from build123d import *

# Parameters (mm, degrees)
BOSS_EXTRUDE1_DEPTH = 70
SKETCH2_R           = 10
CUT_EXTRUDE1_DEPTH  = 20
SKETCH3_R           = 20
CUT_EXTRUDE2_DEPTH  = 71


with BuildPart() as part:
    # Sketch1 → Boss-Extrude1 (new body)
    with BuildSketch(Plane(origin=(0, 0, 0), x_dir=(1, 0, 0), z_dir=(0, 1, 0))):
        with BuildLine():
            Line((0, 100), (600, 100))
            ThreePointArc((600, 100), (700, 0), (600, -100))
            Line((600, -100), (0, -100))
            ThreePointArc((0, -100), (-100, 0), (0, 100))
        make_face()
    extrude(amount=BOSS_EXTRUDE1_DEPTH)

    # Sketch2 → Cut-Extrude1 (cut)
    with BuildSketch(Plane(origin=(0, 70, 0), x_dir=(1, 0, 0), z_dir=(0, 1, 0))):
        Circle(SKETCH2_R)
    extrude(amount=-CUT_EXTRUDE1_DEPTH, mode=Mode.SUBTRACT)

    # Sketch3 → Cut-Extrude2 (cut, through all)
    with BuildSketch(Plane(origin=(0, 70, 0), x_dir=(1, 0, 0), z_dir=(0, 1, 0))):
        with Locations((600, 0)):
            Circle(SKETCH3_R)
    extrude(amount=-CUT_EXTRUDE2_DEPTH, mode=Mode.SUBTRACT)


solid = part.part
Check sheet for the modelled part. Datum: model origin and axes. Units: mm. Round coordinates to 2 decimals unless told otherwise and drop trailing zeros. Order: outer loops, then holes, each group sorted by start corner. A loop starts at its lowest first (then second) coordinate and runs counter-clockwise, first axis right, second up.
Q1. Cross-section at A-A, the plane z = 0. Enter the section's corners in (x, y).
Filled sheet:
outline: (-100, 0) - (580, 0) - (580, 70) - (10, 70) - (10, 50) - (-10, 50) - (-10, 70) - (-100, 70) - close; (620, 0) - (700, 0) - (700, 70) - (620, 70) - close
Q2. Cross-section at B-B, the plane y = 28. Enter the section's corners in (x, z), plus the area to 3 significant figures.
Filled sheet:
outline: (0, -100) - (600, -100) arc R100 ccw to (600, 100) - (0, 100) arc R100 ccw to start; hole circle Ø40 at (600, 0)
area: 150,000 mm2
Q3. Depth check by flat-ended pin: P1, Ø12, axis at x = 603, y = 19.5, coming from the +Z side; P2, Ø8, axis at y = 50.5, z = -5.5, coming from the -X side; P3, Ø16, axis at x = 0, z = 0, coming from the +Y side. Enter the tip coordinate at first touch or a pass-through.
Filled sheet:
P1: stops at z = 100
P2: stops at x = -99.99
P3: stops at y = 50
Q4. Cross-section at C-C, the plane z = 43.5. Enter the section's corners in (x, y).
Filled sheet:
outline: (-90.04, 0) - (690.04, 0) - (690.04, 70) - (-90.04, 70) - close
Q5. Scan lines: L1, parallel to X at y = 62, z = 0; L2, parallel to X at y = 31, z = 0; L3, parallel to Z at x = 0, y = 54. Record each from-to range of solid material in increasing order.
Filled sheet:
L1: x = -100 to -10, 10 to 580, 620 to 700
L2: x = -100 to 580, 620 to 700
L3: z = -100 to -10, 10 to 100
Q6. Draft check along X on faces 1 (the face through (-2.17, 60.14, 9.76)), 2 (the face through (0, 50, 0)), 3 (the face through (296, 35, -100)), 4 (the face through (699.976, 34.51, -2.199)). Enter one of: pulls with the +X half, pulls with the -X half, needs draft (parallel to the pull), parting line crosses it, or undercut.
Filled sheet:
face 1: undercut
face 2: undercut
face 3: needs draft
face 4: pulls with the +X half
Q7. Cross-section at D-D, the plane z = -82.5. Enter the section's corners in (x, y), plus the area to 3 significant figures.
Filled sheet:
outline: (-56.51, 0) - (656.51, 0) - (656.51, 70) - (-56.51, 70) - close
area: 49,900 mm2
